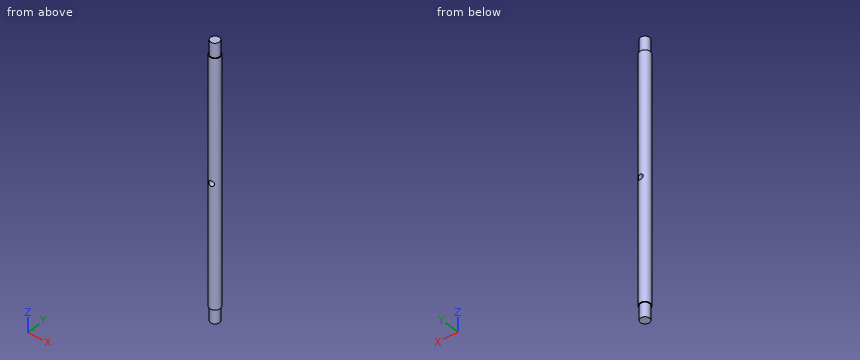
```python
from build123d import *

# Parameters (mm, degrees)
SKETCH1_R                           = 3
BOSS_EXTRUDE1_DEPTH                 = 138
SKETCH2_R                           = 2.5
BOSS_EXTRUDE2_DEPTH                 = 8
BOSS_EXTRUDE3_START                 = 8
SKETCH3_R                           = 2.5
BOSS_EXTRUDE3_DEPTH                 = 8
CUT_EXTRUDE1_REACH                  = 148.062
CUT_EXTRUDE1_END_RADIUS             = 3
SKETCH4_R                           = 1.5
CUT_EXTRUDE1_DIRECTION_2_REACH      = 148.062
CUT_EXTRUDE1_DIRECTION_2_END_RADIUS = 3


with BuildPart() as part:
    # Sketch1 → Boss-Extrude1 (new body)
    with BuildSketch(Plane.XY):
        Circle(SKETCH1_R)
    extrude(amount=BOSS_EXTRUDE1_DEPTH)

    # Sketch2 → Boss-Extrude2 (add)
    with BuildSketch(Plane.XY.offset(138)):
        Circle(SKETCH2_R)
    extrude(amount=BOSS_EXTRUDE2_DEPTH)

    # Sketch3 → Boss-Extrude3 (add)
    with BuildSketch(Plane(origin=(0, 0, 0), x_dir=(-1, 0, 0), z_dir=(0, 0, -1)).offset(BOSS_EXTRUDE3_START)):
        with Locations(Location((0, 0, 0), (0, 0, 180))):
            Circle(SKETCH3_R)
    extrude(amount=-BOSS_EXTRUDE3_DEPTH)

    # Cut-Extrude1: up to this cylinder (the profile starts inside it)
    cut_extrude1_end = Plane(origin=(0, 0, 69), z_dir=(0, 0, -1)) * Cylinder(CUT_EXTRUDE1_END_RADIUS, 303.124, mode=Mode.PRIVATE)
    # Sketch4 → Cut-Extrude1 (cut, up to the surface)
    with BuildSketch(Plane(origin=(0, 0, 0), x_dir=(1, 0, 0), z_dir=(0, 1, 0)), mode=Mode.PRIVATE) as cut_extrude1_sk1:
        with Locations(Location((0.25, -69, 0), (0, 0, 270))):
            Circle(SKETCH4_R)
    cut_extrude1_tool1 = extrude(cut_extrude1_sk1.sketch, amount=-CUT_EXTRUDE1_REACH, mode=Mode.PRIVATE) & cut_extrude1_end
    add(cut_extrude1_tool1.solids().sort_by_distance((0.25, 0, 69))[0], mode=Mode.SUBTRACT)

    # Cut-Extrude1 direction 2: up to this cylinder (the profile starts inside it)
    cut_extrude1_direction_2_end = Plane(origin=(0, 0, 69), z_dir=(0, 0, -1)) * Cylinder(CUT_EXTRUDE1_DIRECTION_2_END_RADIUS, 303.124, mode=Mode.PRIVATE)
    # Sketch4 → Cut-Extrude1 direction 2 (cut, up to the surface)
    with BuildSketch(Plane(origin=(0, 0, 0), x_dir=(1, 0, 0), z_dir=(0, 1, 0)), mode=Mode.PRIVATE) as cut_extrude1_direction_2_sk1:
        with Locations(Location((0.25, -69, 0), (0, 0, 270))):
            Circle(SKETCH4_R)
    cut_extrude1_direction_2_tool1 = extrude(cut_extrude1_direction_2_sk1.sketch, amount=CUT_EXTRUDE1_DIRECTION_2_REACH, mode=Mode.PRIVATE) & cut_extrude1_direction_2_end
    add(cut_extrude1_direction_2_tool1.solids().sort_by_distance((0.25, 0, 69))[0], mode=Mode.SUBTRACT)


solid = part.part
```
CAD build for the part. Positions are in the model's coordinates, mm. Round coordinates to 2 decimals unless told otherwise and drop trailing zeros. Write each loop counter-clockwise with the first axis right and the second up, starting at its lowest first coordinate (ties: lowest second). Pieces come first, ordered by that corner, then holes. Notation, with made-up numbers: (-4.75, 83.5) -> (30.25, 83.5) arc R29 cw to (30.25, 109.5) -> close; hole circle Ø7 at (51.5, 32). An arc over 180 degrees is marked (long way). Answer in a Markdown table with one row per item. Add a question column.
Item 1: Drill centre lines: line 1 (Z direction, x = 0.5, y = -2); line 2 (X direction, y = -0.25, z = 69); line 3 (Y direction, x = -0.25, z = 83). Where is each one in solid material? Low to high. Write a range as from..to.
Item 2: Drop a flat-ended pin along its axis: pin 1 Ø2 at (x, z) = (2.5, 75) entering from +Y. Give the stop position or say it passes through.
Item 3: Saw through at A-A, the plane y = 0. Write the cut outline in (x, z).
Item 4: Saw through at D-D, the plane z = 132.5. Write the cut outline in (x, y), then the cut area to 3 significant figures.
Item 5: Saw through at B-B, the plane x = 0.25. Write the cut outline in (y, z), then the cut area to 3 significant figures.
Item 6: Saw through at C-C, the plane z = 69. Write the cut outline in (x, y), then the cut area to 3 significant figures.
Findings below:
| question | item | result |
|---|---|---|
| 1 | line 1 | z = -8..67.52, 70.48..146 |
| 1 | line 2 | x = -2.99..-1.25, 1.75..2.99 |
| 1 | line 3 | y = -2.99..2.99 |
| 2 | pin 1 | stops at y = 2.6 |
| 3 | outline | (-3, 0) -> (-2.5, 0) -> (-2.5, -8) -> (2.5, -8) -> (2.5, 0) -> (3, 0) -> (3, 138) -> (2.5, 138) -> (2.5, 146) -> (-2.5, 146) -> (-2.5, 138) -> (-3, 138) -> close; hole circle Ø3 at (0.25, 69) |
| 4 | outline | circle Ø6 at (0, 0) |
| 4 | area | 28.3 mm^2 |
| 5 | outline | (-2.99, 0) -> (-2.49, 0) -> (-2.49, -8) -> (2.49, -8) -> (2.49, 0) -> (2.99, 0) -> (2.99, 67.5) -> (-2.99, 67.5) -> close; (-2.99, 70.5) -> (2.99, 70.5) -> (2.99, 138) -> (2.49, 138) -> (2.49, 146) -> (-2.49, 146) -> (-2.49, 138) -> (-2.99, 138) -> close |
| 5 | area | 887 mm^2 |
| 6 | outline | (-1.25, -2.73) -> (-1.25, 2.73) arc R3 ccw to start; (1.75, -2.44) arc R3 ccw to (1.75, 2.44) -> close |
| 6 | area | 11.1 mm^2 |
